The model under review builds one solid part; all positions refer to its coordinate system, in mm. Face numbers are marked on the shaded views. A direction names the side the tool comes from. Coordinates: 2 decimals unless noted, no trailing zeros. Order: outer loops, then holes, each group sorted by start corner. A loop starts at its lowest first (then second) coordinate and runs counter-clockwise, first axis right, second up. Notation, with made-up numbers: (33.25, -34) -> (49.25, -34) arc R18 ccw to (49.25, -16) -> close; hole circle Ø10 at (-8, 74). An arc over 180 degrees is marked (long way). Use one line per item in the form item = value. Start each with the question number.
(1) Take a section at C-C (x = -19). State the section outline as (y, z) points (3 decimals).
(2) Take a section at D-D (x = -4). State the section outline as (y, z) points (3 decimals), then the cut area to 3 significant figures.
(3) For the marked faces 4, 5 and 6, list the 3-axis set-ups (+Z, -Z, +X, -X, +Y, -Y) from which the entire face can be reached by the end or side of a thin tool; tool diameter is ignored.
(4) Take a section at B-B (z = 0). State how many separate pieces and enclosed holes the cut face has, then the cut area to 3 significant figures.
(5) Wall thickness on line 1 along Y through (x, z) = (3, 0) (3 decimals); line 2 along Y through (x, z) = (14.5, -5); line 3 along X through (y, z) = (-81.5, -32.5): over which ranges is each line inside the solid? List them lowest first.
(6) Mouldability with a two-part tool opening along Y and no side actions: class the marked faces 1, 2 and 3 as +Y half, -Y half, draft (parallel to the pull), parting line (faces both ways), or undercut.
(7) Insertion check: pin 1 Ø8 at (x, y) = (10.5, -3) entering from -Z; pin 2 Ø3 at (x, y) = (20, 7) entering from +Z; pin 3 Ø12 at (y, z) = (13.74, 42.27) entering from +X (3 decimals). Each pin has a flat end and moves straight along its axis. Give the tip position at first contact, or say it passes through.
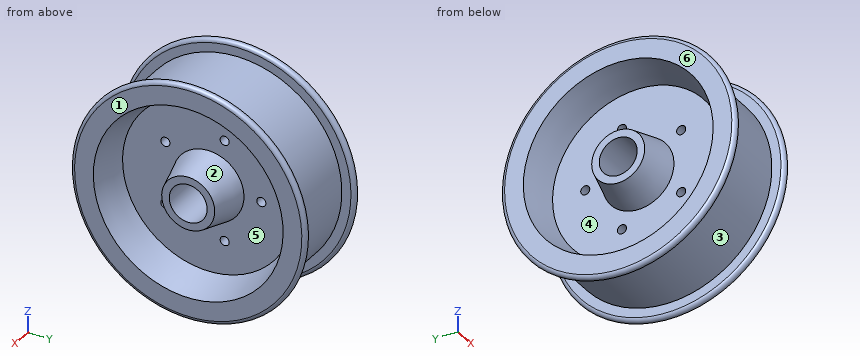
```python
from build123d import *

# Parameters (mm, degrees)
SKETCH2_R          = 3.81
CUT_EXTRUDE1_DEPTH = 148.115947179


with BuildPart() as part:
    # Sketch1 → Revolve1 (revolve)
    with BuildSketch(Plane.XY, mode=Mode.PRIVATE) as revolve1_sk:
        with BuildLine():
            ThreePointArc((-38.1, 95.25), (-34.925, 98.425), (-31.75, 95.25))
            Line((-31.75, 95.25), (-31.75, 87.63))
            Line((-31.75, 87.63), (31.75, 87.63))
            Line((31.75, 87.63), (31.75, 95.25))
            ThreePointArc((31.75, 95.25), (34.925, 98.425), (38.1, 95.25))
            Line((38.1, 95.25), (38.1, 79.5274))
            Line((38.1, 79.5274), (9.525, 71.870751826))
            Line((9.525, 71.870751826), (9.525, 29.881648174))
            Line((9.525, 29.881648174), (38.1, 22.225))
            Line((38.1, 22.225), (38.1, 15.875))
            Line((38.1, 15.875), (-38.1, 15.875))
            Line((-38.1, 15.875), (-38.1, 22.225))
            Line((-38.1, 22.225), (-9.525, 29.881648174))
            Line((-9.525, 29.881648174), (-9.525, 71.870751826))
            Line((-9.525, 71.870751826), (-38.1, 79.5274))
            Line((-38.1, 79.5274), (-38.1, 95.25))
        make_face()
    revolve(revolve1_sk.sketch.rotate(Axis((-74.767669173, 0, 0), (1, 0, 0)), 90), axis=Axis((-74.767669173, 0, 0), (1, 0, 0)))

    # Sketch2 → Cut-Extrude1 (cut, through all)
    with BuildSketch(Plane(origin=(9.525, 0, 0), x_dir=(0, 0, -1), z_dir=(1, 0, 0))):
        with Locations((0, 44.45)):
            Circle(SKETCH2_R)
        with Locations((42.274462149, 13.7358054)):
            Circle(SKETCH2_R)
        with Locations((26.127054464, -35.9608054)):
            Circle(SKETCH2_R)
        with Locations((-26.127054464, -35.9608054)):
            Circle(SKETCH2_R)
        with Locations((-42.274462149, 13.7358054)):
            Circle(SKETCH2_R)
    extrude(amount=-CUT_EXTRUDE1_DEPTH, mode=Mode.SUBTRACT)


solid = part.part
```
Findings:
q1.outline = circle Ø175.26 at (0, 0); circle Ø54.686 at (0, 0); hole circle Ø148.819 at (0, 0); hole circle Ø31.75 at (0, 0)
q2.outline = circle Ø175.26 at (0, 0); hole circle Ø7.62 at (-35.961, -26.127); hole circle Ø7.62 at (-35.961, 26.127); hole circle Ø31.75 at (0, 0); hole circle Ø7.62 at (13.736, -42.274); hole circle Ø7.62 at (13.736, 42.274); hole circle Ø7.62 at (44.45, 0)
q2.area = 23,100 mm²
q3.face_4 = -X
q3.face_5 = +X
q3.face_6 = +Z, -Z, -X, +Y, -Y
q4.separate_pieces = 3
q4.enclosed_holes = 0
q4.area = 5,370 mm²
q5.line_1 = -87.63 to -15.875, 15.875 to 40.64, 48.26 to 87.63
q5.line_2 = -87.49 to -73.03, -28.11 to -15.07, 15.07 to 28.11, 73.03 to 87.49
q5.line_3 = -38.1 to -31.75, 31.75 to 38.1
q6.face_1 = draft
q6.face_2 = undercut
q6.face_3 = parting line
q7.pin_1 = -87.63
q7.pin_2 = 87.46
q7.pin_3 = 9.525
